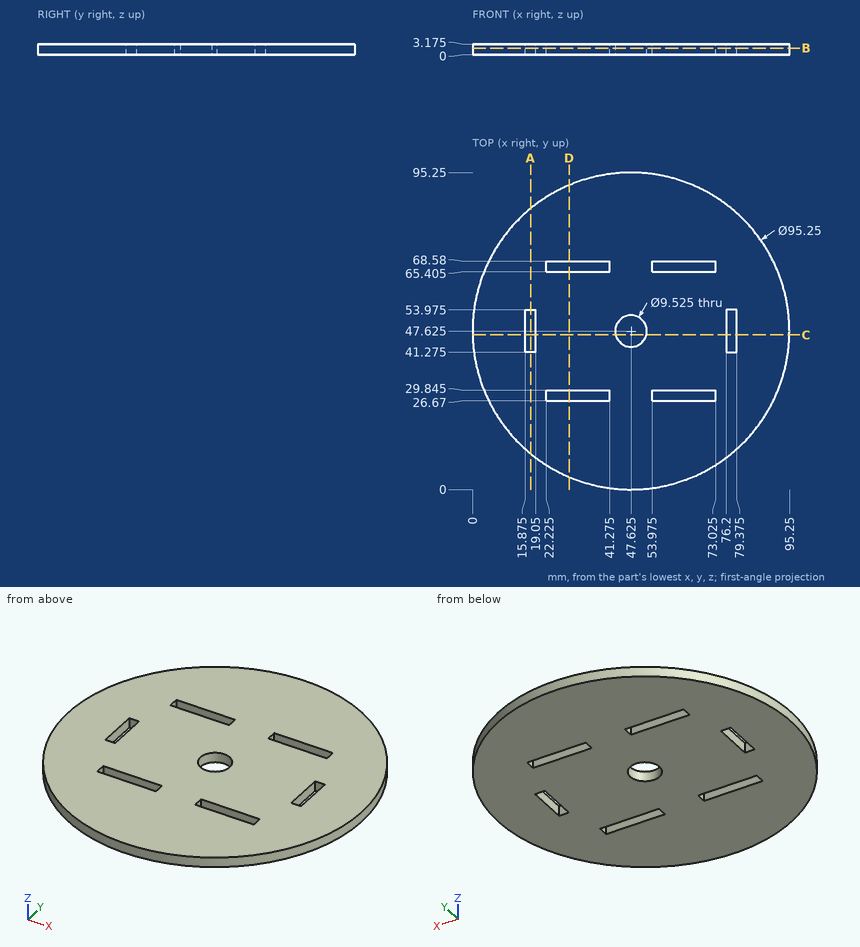
Source: three-view drawing plus pictorial views. Frame: mm from the lowest corner of the part. Coordinates: 2 decimals unless noted, no trailing zeros. Order: outer loops, then holes, each group sorted by start corner. A loop starts at its lowest first (then second) coordinate and runs counter-clockwise, first axis right, second up. Notation, with made-up numbers: (78, 70.5) -> (125, 70.5) arc R20 cw to (125, 87.5) -> close; hole circle Ø7 at (17.25, 24.5). An arc over 180 degrees is marked (long way). Write item = value, one per line.
(1) Line query: line 1 (Y direction, x = 41, z = 3.05) (3 decimals); line 2 (X direction, y = 46.5, z = 2.95) (3 decimals); line 3 (X direction, y = 29.5, z = 2.45) (3 decimals). Output: solid intervals per line, ascending.
Solved:
line_1 = 0.463 to 26.67, 29.845 to 65.405, 68.58 to 94.787
line_2 = 0.013 to 15.875, 19.05 to 42.997, 52.253 to 76.2, 79.375 to 95.237
line_3 = 3.584 to 22.225, 41.275 to 53.975, 73.025 to 91.666
(2) Pin query (flat end, axial travel): pin 1 Ø1.6 at (y, z) = (66.5, 1.5) entering from +X; pin 2 Ø1.6 at (x, z) = (33.5, 2) entering from +Y; pin 3 Ø6 at (x, y) = (76, 85.5) entering from -Z; pin 4 Ø1 at (y, z) = (50, 1) entering from +X. Return the tip coordinate at first contact, or that it passes through.
Solved:
pin_1 = 91.69
pin_2 = 93.35
pin_3 = 0
pin_4 = 95.21
(3) Cut plane C-C on y = 46.5. Return loops of the section in (x, z) (3 decimals).
Solved:
outline = (0.013, 0) -> (15.875, 0) -> (15.875, 3.175) -> (0.013, 3.175) -> close; (19.05, 0) -> (42.997, 0) -> (42.997, 3.175) -> (19.05, 3.175) -> close; (52.253, 0) -> (76.2, 0) -> (76.2, 3.175) -> (52.253, 3.175) -> close; (79.375, 0) -> (95.237, 0) -> (95.237, 3.175) -> (79.375, 3.175) -> close
(4) Cut plane D-D on x = 29. Return loops of the section in (y, z) (3 decimals), plus the area to 3 significant figures.
Solved:
outline = (3.793, 0) -> (26.67, 0) -> (26.67, 3.175) -> (3.793, 3.175) -> close; (29.845, 0) -> (65.405, 0) -> (65.405, 3.175) -> (29.845, 3.175) -> close; (68.58, 0) -> (91.457, 0) -> (91.457, 3.175) -> (68.58, 3.175) -> close
area = 258 mm²
(5) Cut plane B-B on z = 1.9. Count the separate pieces of the cut face and the enclosed holes in it, plus the area to 3 significant figures.
Solved:
separate_pieces = 1
enclosed_holes = 7
area = 6,730 mm²
(6) Cut plane A-A on x = 17.5. Return loops of the section in (y, z) (3 decimals), plus the area to 3 significant figures.
Solved:
outline = (10.738, 0) -> (41.275, 0) -> (41.275, 3.175) -> (10.738, 3.175) -> close; (53.975, 0) -> (84.512, 0) -> (84.512, 3.175) -> (53.975, 3.175) -> close
area = 194 mm²
